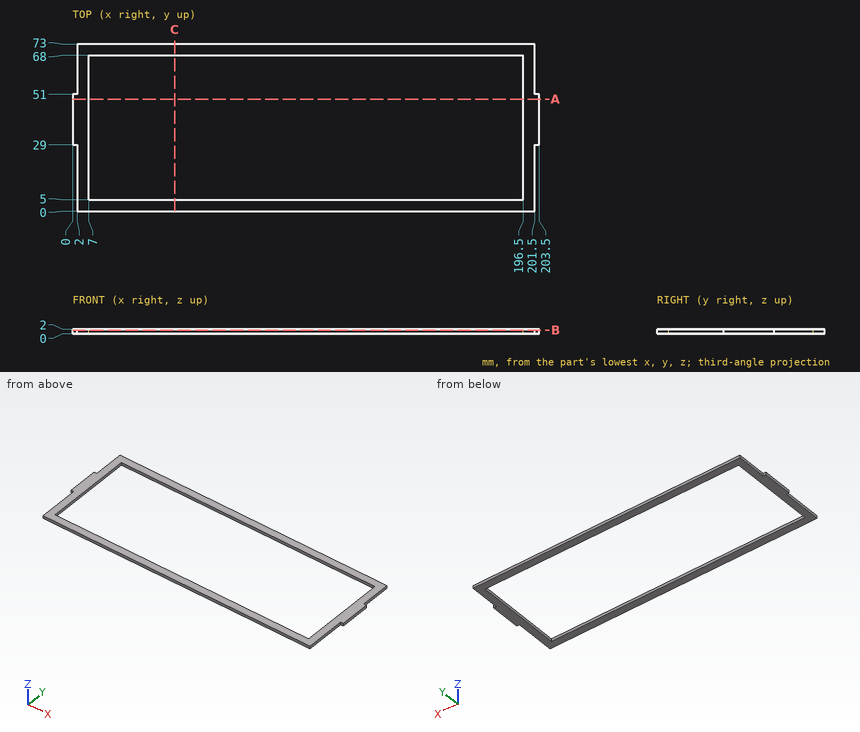
Can you work these out from the drawing? Everything is in mm from the part's minimum corner. Coordinates: 2 decimals unless noted, no trailing zeros. Loops run counter-clockwise (first coordinate to the right, second up) from the corner with the lowest first, then second, coordinate; pieces in that order, holes last.
1. I need wall thicknesses on L1, parallel to X at y = 19.5, z = 1.6; L2, parallel to Y at x = 182.5, z = 1.6; L3, parallel to X at y = 46.5, z = 0.25. Which ranges of each line are inside material? Lowest first, please.
2. Imagine slicing it at A-A, the plane y = 49. Please give me the cut outline in (x, z).
3. For P1, Ø1, axis at y = 19, z = 1, coming from the +X side; P2, Ø0.6, axis at x = 202.5, z = 1, coming from the +Y side; P3, Ø0.6, axis at x = 202.5, z = 1, coming from the -Y side, each with a flat end and sliding along its axis, tell me the tip position at first contact or that it passes through.
4. Imagine slicing it at C-C, the plane x = 44.5. Please give me the cut outline in (y, z), and give its area (3 significant figures).
5. Imagine slicing it at B-B, the plane z = 1.7. Please give me the cut outline in (x, y), and give its area (3 significant figures).
Taken from the geometry:
1. L1: x = 2 to 7, 196.5 to 201.5
1. L2: y = 0 to 5, 68 to 73
1. L3: x = 0 to 7, 196.5 to 203.5
2. outline: (0, 0) - (7, 0) - (7, 2) - (0, 2) - close; (196.5, 0) - (203.5, 0) - (203.5, 2) - (196.5, 2) - close
3. P1: stops at x = 201.5
3. P2: stops at y = 51
3. P3: stops at y = 29
4. outline: (0, 0) - (5, 0) - (5, 2) - (0, 2) - close; (68, 0) - (73, 0) - (73, 2) - (68, 2) - close
4. area: 20.0 mm2
5. outline: (0, 29) - (2, 29) - (2, 0) - (201.5, 0) - (201.5, 29) - (203.5, 29) - (203.5, 51) - (201.5, 51) - (201.5, 73) - (2, 73) - (2, 51) - (0, 51) - close; hole (7, 5) - (196.5, 5) - (196.5, 68) - (7, 68) - close
5. area: 2,710 mm2
